```python
from build123d import *

# Parameters (mm, degrees)
SKETCH1_W           = 130
SKETCH1_H           = 60
SKETCH1_R           = 2.5
SKETCH1_R_2         = 4.499999999
BOSS_EXTRUDE1_DEPTH = 10


with BuildPart() as part:
    # Sketch1 → Boss-Extrude1 (new body)
    with BuildSketch(Plane(origin=(0, 0, 0), x_dir=(0, 0, -1), z_dir=(1, 0, 0))):
        with Locations((3.813160791, 27.897530874)):
            Rectangle(SKETCH1_W, SKETCH1_H)
        with Locations((-36.186839209, 52.897530874)):
            Circle(SKETCH1_R, mode=Mode.SUBTRACT)
        with Locations((-36.186839209, 2.897530874)):
            Circle(SKETCH1_R, mode=Mode.SUBTRACT)
        with Locations((43.813160791, 2.897530874)):
            Circle(SKETCH1_R, mode=Mode.SUBTRACT)
        with Locations((43.813160791, 52.897530874)):
            Circle(SKETCH1_R, mode=Mode.SUBTRACT)
        with Locations((3.813160791, 27.897530874)):
            Circle(SKETCH1_R_2, mode=Mode.SUBTRACT)
        with BuildLine():
            Line((-5.464379102, 30.775341326), (-4.081605515, 33.606305024))
            ThreePointArc((-4.081605515, 33.606305024), (-1.369183898, 34.499769949), (-0.528409533, 31.770555947))
            Line((-0.528409533, 31.770555947), (-1.869576404, 29.020756356))
            ThreePointArc((-1.869576404, 29.020756356), (-4.544523089, 28.10012945), (-5.464379102, 30.775341326))
        make_face(mode=Mode.SUBTRACT)
        with BuildLine():
            Line((5.31316079, 18.397530874), (2.313160791, 18.397530874))
            ThreePointArc((2.313160791, 18.397530874), (0.313160792, 20.397530874), (2.313160791, 22.397530873))
            Line((2.313160791, 22.397530873), (5.31316079, 22.397530873))
            ThreePointArc((5.31316079, 22.397530873), (7.313160789, 20.397530874), (5.31316079, 18.397530874))
        make_face(mode=Mode.SUBTRACT)
        with BuildLine():
            Line((5.31316079, 33.374248764), (2.313160791, 33.374248764))
            ThreePointArc((2.313160791, 33.374248764), (0.31316079, 35.374248765), (2.313160791, 37.374248765))
            Line((2.313160791, 37.374248765), (5.31316079, 37.374248765))
            ThreePointArc((5.31316079, 37.374248765), (7.313160791, 35.374248765), (5.31316079, 33.374248764))
        make_face(mode=Mode.SUBTRACT)
        with BuildLine():
            Line((9.471997672, 29.038205562), (8.081045524, 31.961596177))
            ThreePointArc((8.081045524, 31.961596177), (9.113942414, 34.555839775), (11.733632625, 33.589300054))
            Line((11.733632625, 33.589300054), (13.083423708, 30.758314735))
            ThreePointArc((13.083423708, 30.758314735), (12.137765277, 28.092547131), (9.471997672, 29.038205562))
        make_face(mode=Mode.SUBTRACT)
    extrude(amount=BOSS_EXTRUDE1_DEPTH)


solid = part.part
```
The listing builds one solid part. Answer for the finished solid, in the listing's coordinates (mm). A direction names the side the tool comes from. Round coordinates to 2 decimals unless told otherwise and drop trailing zeros. Loops run counter-clockwise (first coordinate to the right, second up) from the corner with the lowest first, then second, coordinate; pieces in that order, holes last. Notation, with made-up numbers: (63.5, 86.5) - (118.5, 86.5) arc R12 ccw to (118.5, 109.5) - close; hole circle Ø9 at (60, -6.5). An arc over 180 degrees is marked (long way). Return JSON: item names as keys, results as strings. Group by question number.
1. Which of the six approach directions +Z, -Z, +X, -X, +Y, -Y give full straight-line access (tool end or side, diameter ignored) to faces 4 (the flat face through (4.93, 30.479, -8.786)), 5 (the flat face through (5, 27, 61.187))?
2. The mould has two halves that part along Y. Classify faces 1 (the flat face through (5, -2.102, -3)), 2 (the cylindrical face through (4.93, 20.354, -0.314)), 3 (the flat face through (5, 27, -68.813)): pulls with the +Y half, pulls with the -Y half, needs draft (parallel to the pull), parting line crosses it, or undercut.
3. The part is cut by section B-B on x = 3.75. State how many separate pieces and enclosed holes the cut face has, then the cut area to 3 significant figures.
4. The part is cut by section A-A on y = 26.5. Determine the outline of the cut face in (x, z), then the cut area to 3 significant figures.
5. This flat-tipped pin is pushed along its axis until it touches: P1, Ø3, axis at y = 2.9, z = 36.19, coming from the +X side. Where does it stop, or does it pass through?
6. Consider probe 1 along Z at (x, y) = (3, 53); probe 2 along Z at (x, y) = (5.5, 31.5); probe 3 along Z at (x, y) = (7.75, 54). Determine where each line is inside the solid, lowest interval first.
Resolved:
{
 "1": {"face 4": "+X, -X", "face 5": "+Z, +X, -X, +Y, -Y"},
 "2": {"face 1": "pulls with the -Y half", "face 2": "undercut", "face 3": "needs draft"},
 "3": {"separate pieces": "1", "enclosed holes": "9", "area": "7,560 mm²"},
 "4": {"outline": "(0, -68.81) - (10, -68.81) - (10, -8.09) - (0, -8.09) - close; (0, 0.46) - (10, 0.46) - (10, 61.19) - (0, 61.19) - close", "area": "1,210 mm²"},
 "5": {"P1": "passes through"},
 "6": {"probe 1": "z = -68.81 to -46.31, -41.32 to 33.69, 38.68 to 61.19", "probe 2": "z = -68.81 to -12.73, -8.3 to -6.51, -1.12 to 0.66, 5.11 to 61.19", "probe 3": "z = -68.81 to -46.06, -41.57 to 33.94, 38.43 to 61.19"}
}
